Autodesk Inventor part; units mm, degrees
ref_plane "YZ Plane" through (0, 0, 0) normal (1, 0, 0) x (0, 1, 0)
ref_plane "XZ Plane" through (0, 0, 0) normal (0, 1, 0) x (-1, 0, 0)
ref_plane "XY Plane" through (0, 0, 0) normal (0, 0, 1) x (1, 0, 0)
sketch "Sketch1" plane through (0, 0, 0) normal (0, 1, 0) x (-1, 0, 0)
  line L0 (6.793, 18.7845) -> (-263.207, 18.7845)
  line L1 (-263.207, 18.7845) -> (-263.207, -581.2155)
  line L2 (-263.207, -581.2155) -> (6.793, -581.2155)
  line L3 (6.793, -581.2155) -> (6.793, 18.7845)
  point P0 (0, 0)
  dimension "d0" = 270
  dimension "d1" = 600
extrude "Extrusion1" add sketch "Sketch1" along normal blind 10
sketch "Sketch2" plane through (0, 10, 0) normal (0, 1, 0) x (1, 0, 0)
  point P0 (0, 0)
sketch "Sketch3" plane through (0, 10, 0) normal (0, 1, 0) x (1, 0, 0)
  circle A0 centre (131.029, 274.6873) radius 110
  point P0 (0, 0)
  dimension "d4" = 220
extrude "Extrusion2" add sketch "Sketch3" along normal blind 140
sketch "Sketch4" plane through (131.029, 150, -274.6873) normal (0, 1, 0) x (1, 0, 0)
  circle A0 centre (0, 0) radius 110
  line L0 (-75.1726, -80.3062) -> (75.1726, -80.3062)
  line L1 (75.1726, -80.3062) -> (75.1726, 80.3062)
  line L2 (75.1726, 80.3062) -> (-75.1726, 80.3062)
  line L3 (-75.1726, 80.3062) -> (-75.1726, -80.3062)
  line L4 (-75.1726, -80.3062) -> (75.1726, 80.3062) construction
  line L5 (75.1726, -80.3062) -> (-75.1726, 80.3062) construction
  arc A1 (-75.1726, 80.3062) -> (-75.1726, -80.3062) centre (0, 0) ccw
  arc A2 (75.1726, -80.3062) -> (75.1726, 80.3062) centre (0, 0) ccw
  point P0 (-131.029, -274.6873)
  point P1 (-75.1726, 80.3062)
  point P2 (75.1726, -80.3062)
extrude "Extrusion3" cut sketch "Sketch4" against normal blind 92 contours A0 L1 | L1 L0 L3 L2 | L3 A0
sketch "Sketch5" plane through (206.2016, 150, -194.3811) normal (0, 0, -1) x (-1, 0, 0)
  circle A0 centre (72.7519, -41.0963) radius 25
  point P0 (206.2016, -150)
  dimension "d9" = 50
extrude "Extrusion4" cut sketch "Sketch5" against normal blind 92
sketch "Sketch6" plane through (55.8564, 150, -354.9935) normal (0, 0, 1) x (1, 0, 0)
  circle A0 centre (74.775, -43.4815) radius 25
  point P0 (-55.8564, -150)
  dimension "d12" = 50
extrude "Extrusion5" cut sketch "Sketch6" against normal blind 92
Check sheet for the modelled part. Datum: model origin and axes. Units: mm. A direction names the side the tool comes from. Round coordinates to 2 decimals unless told otherwise and drop trailing zeros. Write each loop counter-clockwise with the first axis right and the second up, starting at its lowest first coordinate (ties: lowest second). Pieces come first, ordered by that corner, then holes. Notation, with made-up numbers: M 74.25,54 L 118.25,54 A13 cw 118.25,77 Z; hole C 43.25,77.5 d11. An arc over 180 degrees is marked long. Write item = value, one per line. Start each with the question number.
1. Gauge pin test, flat ends, axial feed: pin 1 (4 mm diameter, centred on x = 138, z = -467, fed in from +Y); pin 2 (8 mm diameter, centred on y = 55, z = -353.5, fed in from +X); pin 3 (10 mm diameter, centred on x = 81.5, y = 96.5, fed in from -Z). Record the tip position at first contact, or that the pin passes through.
2. Scan lines: line 1 (Z direction, x = 127, y = 74); line 2 (Y direction, x = 92, z = -343); line 3 (Y direction, x = 147, z = -480). Record each from-to range of solid material in increasing order. Write a range as [from, to].
3. Section check B-B, the plane z = -179.5. Record the cut outline in (x, y).
4. Tool access check on faces 5 (the flat face through (130, 150, -183)), 6 (the cylindrical face through (232.64, 47.91, -316.82)), 7 (the flat face through (149, 84, -354.994)). Record the directions out of +Z, -Z, +X, -X, +Y, -Y that give a thin tool (end or side, any length) a straight path to the whole face; none if there is none.
5. Section check D-D, the plane y = 51. Record the cut outline in (x, z).
6. Section check C-C, the plane z = -55.5. Record the cut outline in (x, y).
7. Release check for a two-part mould opening along Y. For faces 1 (the flat face through (129, 58, -276)), 2 (the flat face through (113, 84, -194.381)), 3 (the cylindrical face through (127.377, 131.306, -369.634)), 4 (the cylindrical face through (109.6, 116.4, -179.7)) record: pulls with the +Y half, pulls with the -Y half, needs draft (parallel to the pull), parting line crosses it, or undercut.
8. Section check A-A, the plane x = 230. Record the cut outline in (y, z).
Results found:
q1.pin_1 = 10
q1.pin_2 = 211.67
q1.pin_3 = -375.27
q2.line_1 = [-384.61, -354.99], [-194.38, -164.76]
q2.line_2 = [0, 58]
q2.line_3 = [0, 10]
q3.outline = M -6.79,0 L 263.21,0 L 263.21,10 L 186.16,10 L 186.16,150 L 75.9,150 L 75.9,10 L -6.79,10 Z; hole C 133.45,108.9 d50
q4.face_5 = +Z, -Z, +X, -X, +Y
q4.face_6 = +Y
q4.face_7 = +X, -X, +Y
q5.outline = C 131.03,-274.69 d220
q6.outline = M -6.79,0 L 263.21,0 L 263.21,10 L -6.79,10 Z
q7.face_1 = pulls with the +Y half
q7.face_2 = needs draft
q7.face_3 = undercut
q7.face_4 = undercut
q8.outline = M 0,-581.22 L 10,-581.22 L 10,-322.7 L 58,-322.7 L 58,-226.68 L 10,-226.68 L 10,18.78 L 0,18.78 Z
